Read the model definition and answer for the solid it produces. Units are mm, in the model's axes. Face numbers are marked on the shaded views. A direction names the side the tool comes from. Coordinates: 2 decimals unless noted, no trailing zeros. Order: outer loops, then holes, each group sorted by start corner. A loop starts at its lowest first (then second) coordinate and runs counter-clockwise, first axis right, second up. Notation, with made-up numbers: M 4.5,3 L 9.5,3 A31 cw 9.5,34 Z; hole C 21,59.5 d4. An arc over 180 degrees is marked long. One line per question, with ' | ' between items. Start each with the question number.
1) A tool of negligible diameter and unlimited length cuts with its end or side. For the marked faces 1, 2 and 3, from which of +Z, -Z, +X, -X, +Y, -Y can it reach the whole face along a straight path? Write none if from no direction.
2) Find section A-A, the plane y = 11. Write down the section's boundary in (x, z).
3) Find section D-D, the plane y = 7.5. Write down the section's boundary in (x, z).
4) Find section B-B, the plane x = 3.5. Write down the section's boundary in (y, z), plus the area to 3 significant figures.
5) Consider probe 1 along Z at (x, y) = (-7.75, 10.75); probe 2 along X at (y, z) = (3, 41.65); probe 3 along Z at (x, y) = (13.25, 4). Determine where each line is inside the solid, lowest interval first.
6) Given P1, Ø7, axis at y = 7, z = 1.5, coming from the +X side; P2, Ø5, axis at x = 10, z = 11.5, coming from the +Y side; P3, Ø3.5, axis at x = 10.5, y = 5, coming from the -Z side, each flat-ended and moving along its own axis, determine where each tip first touches the part or whether it passes through.
7) Find section C-C, the plane z = 15. Write down the section's boundary in (x, y), plus the area to 3 significant figures.
8) The mould has two halves that part along Z. Classify the marked faces 4, 5 and 6: +Z half, -Z half, draft (parallel to the pull), parting line (faces both ways), or undercut.
from build123d import *

# Parameters (mm, degrees)
SKETCH_5_W          = 26.8
SKETCH_5_H          = 42.2
SKETCH_5_R          = 1.1
SKETCH_5_W_2        = 12.8
SKETCH_5_H_2        = 23.2
EXTRUDE_1_DEPTH     = 3
SKETCH_7_W          = 9.5
SKETCH_7_H          = 15
SKETCH_7_H_2        = 12.5
EXTRUDE_2_DEPTH     = 17.3
SKETCH_10_R         = 1.75
CUT_EXTRUDE_2_DEPTH = 10
EXTRUDE_START       = -42.2
EXTRUDE_3_DEPTH     = 42.2
SKETCH_16_W         = 15.5
SKETCH_16_H         = 14.7
CUT_EXTRUDE_3_DEPTH = 17.3
FILLET_1_R          = 1
SKETCH_20_W         = 26.8
SKETCH_20_H         = 6
EXTRUDE_5_DEPTH     = 25
SKETCH_21_R         = 2.5
CUT_EXTRUDE_6_DEPTH = 4
SKETCH_22_R         = 1.1
CUT_EXTRUDE_7_DEPTH = 63.361606779


with BuildPart() as part:
    # 草图5 → 凸台-拉伸1 (new body)
    with BuildSketch(Plane(origin=(0, 0, 0), x_dir=(1, 0, 0), z_dir=(0, 1, 0))):
        with Locations((3.4, -11.1)):
            Rectangle(SKETCH_5_W, SKETCH_5_H)
        with Locations(Location((5.9, 2.3, 0), (0, 0, 270))):
            Circle(SKETCH_5_R, mode=Mode.SUBTRACT)
        with Locations(Location((5.9, -24.5, 0), (0, 0, 270))):
            Circle(SKETCH_5_R, mode=Mode.SUBTRACT)
        with Locations((5.9, -11.1)):
            Rectangle(SKETCH_5_W_2, SKETCH_5_H_2, mode=Mode.SUBTRACT)
    extrude(amount=EXTRUDE_1_DEPTH)

    # 草图7 → 凸台-拉伸2 (add)
    with BuildSketch(Plane(origin=(0, 3, 0), x_dir=(1, 0, 0), z_dir=(0, 1, 0))):
        with Locations((-5.25, 2.5)):
            Rectangle(SKETCH_7_W, SKETCH_7_H)
        with Locations((-5.25, -25.95)):
            Rectangle(SKETCH_7_W, SKETCH_7_H_2)
    extrude(amount=EXTRUDE_2_DEPTH)

    # 草图10 → 切除-拉伸2 (cut)
    with BuildSketch(Plane.XY.offset(5)):
        with Locations((-5.25, 11)):
            Circle(SKETCH_10_R)
    extrude(amount=-CUT_EXTRUDE_2_DEPTH, mode=Mode.SUBTRACT)

    # 草图13 → 凸台-拉伸3 (add)
    with BuildSketch(Plane.XY.offset(32.2).offset(EXTRUDE_START)):
        Polygon((-0.5, 20.3), (2.5, 20.3), (2.5, 18.3), (-0.5, 14.3), (-0.5, 15.553856002), align=None)
        Polygon((-10, 15.553856002), (-10, 14.3), (-13, 18.3), (-13, 20.3), (-10, 20.3), align=None)
    extrude(amount=EXTRUDE_3_DEPTH)

    # 草图16 → 切除-拉伸3 (cut)
    with BuildSketch(Plane(origin=(0, 20.3, 0), x_dir=(1, 0, 0), z_dir=(0, 1, 0))):
        with Locations((-5.25, -12.35)):
            Rectangle(SKETCH_16_W, SKETCH_16_H)
    extrude(amount=-CUT_EXTRUDE_3_DEPTH, mode=Mode.SUBTRACT)

    # 圆角1
    fillet_1_edges = [part.edges().sort_by_distance(p)[0] for p in [
        (-13, 20.3, 25.95),
        (2.5, 20.3, 25.95),
        (2.5, 20.3, -2.5),
        (-13, 20.3, -2.5),
    ]]
    fillet(fillet_1_edges, radius=FILLET_1_R)

    # 草图20 → 凸台-拉伸5 (add)
    with BuildSketch(Plane.XY.offset(32.2)):
        with Locations((3.4, 3)):
            Rectangle(SKETCH_20_W, SKETCH_20_H)
    extrude(amount=EXTRUDE_5_DEPTH)

    # 草图21 → 切除-拉伸6 (cut)
    with BuildSketch(Plane(origin=(0, 6, 0), x_dir=(1, 0, 0), z_dir=(0, 1, 0))):
        with Locations(Location((7.15, -47.75, 0), (0, 0, 270))):
            Circle(SKETCH_21_R)
        with Locations(Location((-0.35, -41.65, 0), (0, 0, 270))):
            Circle(SKETCH_21_R)
    extrude(amount=-CUT_EXTRUDE_6_DEPTH, mode=Mode.SUBTRACT)

    # 草图22 → 切除-拉伸7 (cut, through all)
    with BuildSketch(Plane(origin=(0, 2, 0), x_dir=(1, 0, 0), z_dir=(0, 1, 0))):
        with Locations(Location((-0.35, -41.65, 0), (0, 0, 270))):
            Circle(SKETCH_22_R)
        with Locations(Location((7.15, -47.75, 0), (0, 0, 270))):
            Circle(SKETCH_22_R)
    extrude(amount=-CUT_EXTRUDE_7_DEPTH, mode=Mode.SUBTRACT)


solid = part.part
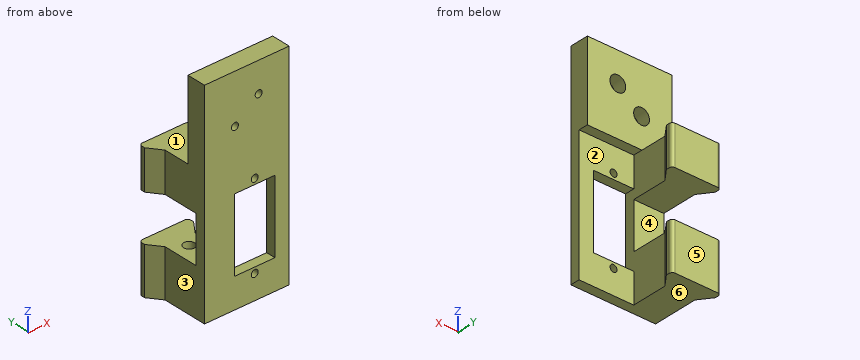
Report:
1) face 1: +Z, +X, -X, +Y | face 2: -Z, +X | face 3: +Z, -Z, -X, -Y
2) outline: M -10,-10 L -0.5,-10 L -0.5,5 L -3.5,5 L -3.5,-5 L -7,-5 L -7,5 L -10,5 Z; M -10,19.7 L -0.5,19.7 L -0.5,32.2 L -10,32.2 Z
3) outline: M -10,-10 L -0.5,-10 L -0.5,5 L -10,5 Z; M -10,19.7 L -0.5,19.7 L -0.5,32.2 L -10,32.2 Z
4) outline: M 0,-10 L 3,-10 L 3,-0.5 L 0,-0.5 Z; M 0,22.7 L 3,22.7 L 3,32.2 L 6,32.2 L 6,57.2 L 0,57.2 Z | area: 207 mm^2
5) probe 1: z = -10 to 5, 19.7 to 32.2 | probe 2: x = -10 to -2.85, 2.15 to 16.8 | probe 3: z = 32.2 to 57.2
6) P1: stops at x = -0.5 | P2: stops at y = 3 | P3: stops at z = 32.2
7) outline: M -10,0 L -0.5,0 L -0.5,3 L -10,3 Z; M 12.3,0 L 16.8,0 L 16.8,3 L 12.3,3 Z | area: 42.0 mm^2
8) face 4: undercut | face 5: draft | face 6: -Z half
